```python
from build123d import *

# Parameters (mm, degrees)
F1_DEPTH     = 3
F0_R         = 1.5
F2_DEPTH     = 2.5
F3_R         = 1.5
F4_DEPTH     = 5.5
F5_DEPTH     = 3
F6_R         = 1.5
F7_DEPTH     = 5.5
F8_DEPTH     = 3
F10_DEPTH    = 5
F11_T4_DEPTH = 32.8926942089
F14_DEPTH    = 0.3
F15_R        = 0.29999
F16_R        = 1
F17_R        = 0.2
F18_DEPTH    = 1
F19_DEPTH    = 1
F20_DEPTH    = 1
F21_R        = 1.5
F22_DEPTH    = 2.5
F23_DEPTH    = 1
F24_DEPTH    = 0.05
F26_DEPTH    = 0.6
F27_SIZE     = 0.3


# Not quite as in the source:
# - a fillet or chamfer that OpenCascade refuses, or shapes differently, is made with other operations: its cross-section is extruded or revolved along the edge and cut away or added
# - a fillet or chamfer is up to 0.001 mm smaller than in the source, because OpenCascade refuses the exact size


with BuildPart() as f1:
    # F0 (on Front) → F1 (new body)
    with BuildSketch(Plane.XZ):
        Polygon((15.2273818341, 37.2200216049), (7.2273818341, 37.2200216049), (7.2273818341, 34.2200216049), (12.2273818341, 29.2200216049), (15.2273818341, 29.2200216049), align=None)
    extrude(amount=F1_DEPTH)

    # F0 (on Front) → F2 (join)
    with BuildSketch(Plane.XZ):
        Polygon((7.2273818341, 34.2200216049), (7.2273818341, 37.2200216049), (0.2273818341, 37.2200216049), (0.2273818341, 26.2200216049), (4.2273818341, 22.2200216049), (15.2273818341, 22.2200216049), (15.2273818341, 29.2200216049), (12.2273818341, 29.2200216049), align=None)
        with Locations((5.2273818341, 27.2200216049)):
            Circle(F0_R, mode=Mode.SUBTRACT)
        Polygon((15.2273818341, 37.2200216049), (7.2273818341, 37.2200216049), (7.2273818341, 34.2200216049), (12.2273818341, 29.2200216049), (15.2273818341, 29.2200216049), align=None)
    extrude(amount=-F2_DEPTH)

    # F3 (on face) → F4 (join)
    with BuildSketch(Plane.XY.offset(37.2200216049)):
        Polygon((0.2273818341, 2.5), (9.7273818341, 2.5), (12.2273818341, 5), (12.2273818341, 12), (4.2273818341, 12), (0.2273818341, 8), align=None)
        with Locations((5.2273818341, 7)):
            Circle(F3_R, mode=Mode.SUBTRACT)
        Polygon((9.7273818341, 2.5), (15.2273818341, 2.5), (15.2273818341, 5), (12.2273818341, 5), align=None)
    extrude(amount=-F4_DEPTH)

    # F3 (on face) → F5 (cut)
    with BuildSketch(Plane.XY.offset(37.2200216049)):
        Polygon((0.2273818341, 2.5), (9.7273818341, 2.5), (12.2273818341, 5), (12.2273818341, 12), (4.2273818341, 12), (0.2273818341, 8), align=None)
        with Locations((5.2273818341, 7)):
            Circle(F3_R, mode=Mode.SUBTRACT)
        Polygon((0.2273818341, 0), (7.2273818341, 0), (9.7273818341, 2.5), (0.2273818341, 2.5), align=None)
    extrude(amount=-F5_DEPTH, mode=Mode.SUBTRACT)

    # F6 (on face) → F7 (join)
    with BuildSketch(Plane.YZ.offset(15.2273818341)):
        Polygon((5, 34.2200216049), (0, 29.2200216049), (0, 22.2200216049), (8, 22.2200216049), (12, 26.2200216049), (12, 34.2200216049), align=None)
        with Locations((7, 27.2200216049)):
            Circle(F6_R, mode=Mode.SUBTRACT)
    extrude(amount=-F7_DEPTH)

    # F6 (on face) → F8 (cut)
    with BuildSketch(Plane.YZ.offset(15.2273818341)):
        Polygon((2.5, 31.7200216049), (0, 29.2200216049), (0, 22.2200216049), (2.5, 22.2200216049), align=None)
        Polygon((5, 31.7200216049), (2.5, 31.7200216049), (2.5, 22.2200216049), (8, 22.2200216049), (12, 26.2200216049), (12, 34.2200216049), (5, 34.2200216049), align=None)
        with Locations((7, 27.2200216049)):
            Circle(F6_R, mode=Mode.SUBTRACT)
        Polygon((5, 34.2200216049), (2.5, 31.7200216049), (5, 31.7200216049), align=None)
    extrude(amount=-F8_DEPTH, mode=Mode.SUBTRACT)

    # F9 (on face) → F10 (cut)
    with BuildSketch(Plane.XZ.offset(3)):
        Polygon((15.2273818341, 32.2200216049), (15.2273818341, 37.2200216049), (10.2273818341, 37.2200216049), align=None)
    extrude(amount=-F10_DEPTH, mode=Mode.SUBTRACT)

    # F11: chamfer of 5 x 3.5533150469 on 1 edges, made by hand


with BuildPart() as f11_tool2:
    # F11_s3 → F11_t4 (new body)
    with BuildSketch(Plane(origin=(-22.6256434487, 0, 22.6256434487), x_dir=(0, 1, 0), z_dir=(0.7071067812, 0, -0.7071067812))):
        Polygon((2, 37.1036957683), (-3, 33.5503807214), (2, 33.5503807214), align=None)
    extrude(amount=F11_T4_DEPTH)

    split(bisect_by=Plane.YZ.offset(15.2273818341), keep=Keep.BOTTOM)

    split(bisect_by=Plane.XZ.offset(3), keep=Keep.BOTTOM)

    split(bisect_by=Plane.XY.offset(37.2200216049), keep=Keep.BOTTOM)


with BuildPart() as f1_1:
    add(f1.part)

    # F11_t1: union F11_tool2
    add(f11_tool2.part)

    # F13 (on 3pt) → F14 (cut, symmetric)
    with BuildSketch(Plane(origin=(13.8158011463, -13.8158011463, 13.8158011463), x_dir=(0.8164965809, 0.4082482905, -0.4082482905), z_dir=(0.5773502692, -0.5773502692, 0.5773502692))):
        Polygon((-1.0654091424, 19.1374719877), (-1.0654091424, 29.2569466706), (-9.8291312908, 24.1972093292), align=None)
        Polygon((-1.9454084062, 20.6616754232), (-8.0691327632, 24.1972093292), (-1.9454084062, 27.7327432351), align=None, mode=Mode.SUBTRACT)
        Polygon((-1.9454084062, 27.7327432351), (-8.0691327632, 24.1972093292), (-1.9454084062, 20.6616754232), align=None)
        Polygon((-7.6691327632, 24.1972093292), (-2.1454084062, 27.3863330736), (-2.1454084062, 21.0080855847), align=None, mode=Mode.SUBTRACT)
    extrude(amount=F14_DEPTH, both=True, mode=Mode.SUBTRACT)

    # F15 (radius 0.3 in the source; OpenCascade refuses exactly that, so slightly less here)
    f15_edges = [f1_1.edges().sort_by_distance(p)[0] for p in [
        (9.635826, 2.591555, 33.883517),
        (11.890877, 2.591555, 31.628466),
        (9.982237, 2.245145, 34.229927),
        (12.237288, 2.245145, 31.974876),
        (9.635826, 0.336504, 31.628466),
        (9.982237, -0.009906, 31.974876),
    ]]
    fillet(f15_edges, radius=F15_R)

    # F16
    f16_edges = [f1_1.edges().sort_by_distance(p)[0] for p in [
        (12.746997, 2.5, 31.720022),
        (9.727382, -0.519615, 31.720022),
        (9.727382, 2.5, 34.739637),
    ]]
    fillet(f16_edges, radius=F16_R)

    # F17
    f17_edges = [f1_1.edges().sort_by_distance(p)[0] for p in [
        (9.467574, 0, 31.460214),
        (12.227382, 2.759808, 31.460214),
        (9.467574, 2.759808, 34.220022),
    ]]
    fillet(f17_edges, radius=F17_R)

    # F18 (add): a face of the model
    f18_faces = [f1_1.faces().sort_by_distance(p)[0] for p in [
        (4.9773818341, 2.5, 31.5856713165),
    ]]
    extrude(f18_faces, amount=F18_DEPTH)

    # F19 (add): a face of the model
    f19_faces = [f1_1.faces().sort_by_distance(p)[0] for p in [
        (9.7273818341, 7.75, 31.592546117),
    ]]
    extrude(f19_faces, amount=F19_DEPTH)

    # F20 (add): a face of the model
    f20_faces = [f1_1.faces().sort_by_distance(p)[0] for p in [
        (4.4773818341, 3.6202081528, 31.7200216049),
    ]]
    extrude(f20_faces, amount=F20_DEPTH)

    # F21 (on face) → F22 (cut)
    with BuildSketch(Plane(origin=(0, 0, 30.7200216049), x_dir=(1, 0, 0), z_dir=(0, 0, -1))):
        Polygon((2.0765037567, -7.8442752363), (4.3831065978, -10.1508780774), (5.0592546763, -9.9697047458), (4.9816089627, -9.679926998), (6.7801908833, -9.1979984248), (6.8578365969, -9.4877761727), (7.5339846753, -9.3066028411), (8.3782599116, -6.1557247637), (6.0716570704, -3.8491219226), (2.920778993, -4.6933971589), (2.7396056614, -5.3695452373), (3.0293834093, -5.4471909508), (2.5474548362, -7.2457728714), (2.2576770883, -7.1681271579), align=None)
        with Locations((5.2273818341, -7)):
            Circle(F21_R, mode=Mode.SUBTRACT)
        Polygon((2.7396056614, -5.3695452373), (2.2576770883, -7.1681271579), (2.5474548362, -7.2457728714), (3.0293834093, -5.4471909508), align=None)
        Polygon((4.9816089627, -9.679926998), (5.0592546763, -9.9697047458), (6.8578365969, -9.4877761727), (6.7801908833, -9.1979984248), align=None)
    extrude(amount=-F22_DEPTH, mode=Mode.SUBTRACT)

    # F21 (on face) → F23 (cut)
    with BuildSketch(Plane(origin=(0, 0, 30.7200216049), x_dir=(1, 0, 0), z_dir=(0, 0, -1))):
        Polygon((0.7242075999, -7.4819285731), (2.0765037567, -7.8442752363), (2.2576770883, -7.1681271579), (1.5815290099, -6.9869538263), (2.063457583, -5.1883719057), (2.7396056614, -5.3695452373), (2.920778993, -4.6933971589), (1.5684828362, -4.3310504957), align=None)
        Polygon((5.0592546763, -9.9697047458), (4.3831065978, -10.1508780774), (4.745453261, -11.5031742342), (7.8963313384, -10.6588989979), (7.5339846753, -9.3066028411), (6.8578365969, -9.4877761727), (7.0390099284, -10.1639242511), (5.2404280078, -10.6458528242), align=None)
    extrude(amount=-F23_DEPTH, mode=Mode.SUBTRACT)

    # F21 (on face) → F24 (join, symmetric)
    with BuildSketch(Plane(origin=(0, 0, 30.7200216049), x_dir=(1, 0, 0), z_dir=(0, 0, -1))):
        Polygon((1.5815290099, -6.9869538263), (2.2576770883, -7.1681271579), (2.7396056614, -5.3695452373), (2.063457583, -5.1883719057), align=None)
        Polygon((6.8578365969, -9.4877761727), (5.0592546763, -9.9697047458), (5.2404280078, -10.6458528242), (7.0390099284, -10.1639242511), align=None)
    extrude(amount=F24_DEPTH, both=True)

    # F25 (on face) → F26 (join)
    with BuildSketch(Plane(origin=(0, 0, 30.6700216049), x_dir=(1, 0, 0), z_dir=(0, 0, -1))):
        Polygon((2.7396056614, -5.3695452373), (2.2576770883, -7.1681271579), (2.7406400014, -7.2975366804), (3.2225685746, -5.4989547598), align=None)
        Polygon((1.5815290099, -6.9869538263), (2.2576770883, -7.1681271579), (2.7396056614, -5.3695452373), (2.063457583, -5.1883719057), align=None)
        Polygon((4.9298451537, -9.4867418327), (5.0592546763, -9.9697047458), (6.8578365969, -9.4877761727), (6.7284270743, -9.0048132595), align=None)
        Polygon((5.0592546763, -9.9697047458), (5.2404280078, -10.6458528242), (7.0390099284, -10.1639242511), (6.8578365969, -9.4877761727), align=None)
    extrude(amount=F26_DEPTH)

    # F27
    f27_edges = [f1_1.edges().sort_by_distance(p)[0] for p in [
        (2.981604, 6.398246, 30.070022),
        (5.829136, 9.245778, 30.070022),
    ]]
    chamfer(f27_edges, length=F27_SIZE)


solid = f1_1.part
```
The listing builds one solid part. Answer for the finished solid, in the listing's coordinates (mm). A direction names the side the tool comes from. Round coordinates to 2 decimals unless told otherwise and drop trailing zeros. Loops run counter-clockwise (first coordinate to the right, second up) from the corner with the lowest first, then second, coordinate; pieces in that order, holes last. Notation, with made-up numbers: (-3.5, 16) - (4.5, 16) arc R16 ccw to (4.5, 37) - close; hole circle Ø8 at (39.25, 29). An arc over 180 degrees is marked (long way). Return JSON: item names as keys, results as strings. Group by question number.
1. The part is cut by section B-B on x = 5.75. Determine the outline of the cut face in (y, z).
2. Which of the six approach directions +Z, -Z, +X, -X, +Y, -Y give full straight-line access (tool end or side, diameter ignored) to faces 1 (the cylindrical face through (12.013, 2.538, 31.609)), 2 (the flat face through (2.7, 6.3, 30.67)), 3 (the flat face through (14.161, 2.535, 31.755)), 4 (the flat face through (9.69, -1.9, 31.76)), 5 (the flat face through (3.21, 8.98, 31.95))?
3. Consider probe 1 along X at (y, z) = (7, 33.75); probe 2 along X at (y, z) = (11.75, 29.25); probe 3 along Y at (x, z) = (10.75, 28.5). Determine where each line is inside the solid, lowest interval first.
4. Each of these flat-tipped pins is pushed along its axis until it touches: P1, Ø1.1, axis at x = 1.5, y = 5.5, coming from the -Z side; P2, Ø6, axis at x = 5.5, y = 5, coming from the +Z side; P3, Ø2.5, axis at x = 5.23, z = 27.22, coming from the -Y side; P4, Ø1.5, axis at y = -1, z = 35.5, coming from the -X side. Where does it stop, or does it pass through?
5. The part is cut by section A-A on z = 28. Determine the outline of the cut face in (x, y), then the cut area to 3 significant figures.
6. The part is cut by section D-D on x = 12.75. Determine the outline of the cut face in (y, z), then the cut area to 3 significant figures.
7. The mould has two halves that part along Z. Classify faces 6 (the cylindrical face through (4.902, 1.726, 25.756)), 7 (the flat face through (13.682, -1.03, 35.745)), 8 (the flat face through (7.95, 7.75, 31.95)), 9 (the flat face through (6, 11, 31.72)): pulls with the +Z half, pulls with the -Z half, needs draft (parallel to the pull), parting line crosses it, or undercut.
8. The part is cut by section C-C on y = -1.25. Determine the outline of the cut face in (x, z).
Resolved:
{
 "1": {"outline": "(0, 22.22) - (3.5, 22.22) - (3.5, 25.81) - (0, 25.81) - close; (0, 28.63) - (3.5, 28.63) - (3.5, 30.72) - (3.94, 30.72) - (3.94, 33.22) - (5.59, 33.22) - (5.59, 34.22) - (0, 34.22) - close; (8.41, 33.22) - (9.78, 33.22) - (9.78, 30.67) - (9.27, 30.67) - (9.27, 30.37) - (9.58, 30.07) - (10.51, 30.07) - (10.51, 31.72) - (11.23, 31.72) - (11.23, 30.72) - (12, 30.72) - (12, 34.22) - (8.41, 34.22) - close"},
 "2": {"face 1": "none", "face 2": "+Y", "face 3": "-Z, +X, +Y", "face 4": "-Z, -X, -Y", "face 5": "-Z"},
 "3": {"probe 1": "x = 0.23 to 3.73, 6.73 to 12.23", "probe 2": "x = 8.73 to 12.23", "probe 3": "y = 0 to 6.22, 7.78 to 12"},
 "4": {"P1": "stops at z = 30.07", "P2": "stops at z = 34.22", "P3": "passes through", "P4": "stops at x = 7.23"},
 "5": {"outline": "(0.23, 0) - (3.95, 0) - (3.95, 3.5) - (0.23, 3.5) - close; (6.51, 0) - (12.23, 0) - (12.23, 5.72) - (8.73, 5.72) - (8.73, 3.5) - (6.51, 3.5) - close; (8.73, 8.28) - (12.23, 8.28) - (12.23, 12) - (8.73, 12) - close", "area": "53.8 mm²"},
 "6": {"outline": "(-3, 29.22) - (-0.07, 29.22) - (5, 34.29) - (5, 37.22) - (-0.49, 37.22) - (-3, 34.7) - close", "area": "48.0 mm²"},
 "7": {"face 6": "undercut", "face 7": "pulls with the +Z half", "face 8": "needs draft", "face 9": "pulls with the -Z half"},
 "8": {"outline": "(7.23, 34.22) - (12.23, 29.22) - (15.23, 29.22) - (15.23, 33.98) - (11.99, 37.22) - (7.23, 37.22) - close"}
}
